from build123d import *

# Parameters (mm, degrees)
BOSS_EXTRUDE1_DEPTH                      = 3
MIRROR1_AT_THE_SECOND_PLANE_COPY_1_DEPTH = 3
SKETCH2_R                                = 8.5
SKETCH2_R_2                              = 4.75
CUT_EXTRUDE1_DEPTH                       = 108.522090753
SKETCH3_R                                = 1.6
CUT_EXTRUDE2_DEPTH                       = 108.522090753
CHAMFER1_SIZE                            = 1.5


with BuildPart() as part:
    # Sketch1 → Boss-Extrude1 (new body)
    with BuildSketch(Plane(origin=(0, 0, 0), x_dir=(1, 0, 0), z_dir=(0, 1, 0))):
        Polygon((-76, -73), (-59.111111111, -73), (-59.111111111, -76), (-42.222222222, -76), (-42.222222222, -73), (-25.333333333, -73), (-25.333333333, -76), (-8.444444444, -76), (-8.444444444, -73), (0, -73), (0, 0), (-76, 0), (-76, -8.444444444), (-73, -8.444444444), (-73, -25.333333333), (-76, -25.333333333), (-76, -42.222222222), (-73, -42.222222222), (-73, -59.111111111), (-76, -59.111111111), align=None)
    boss_extrude1 = extrude(amount=BOSS_EXTRUDE1_DEPTH)



with BuildPart() as mirror1_1:
    # Mirror1: Boss-Extrude1 across plane
    add(boss_extrude1.mirror(Plane(origin=(0, 0, 0), x_dir=(0, 0, 1), z_dir=(1, 0, 0))))


with BuildPart() as part_1:
    add(part.part)

    add(mirror1_1.part)  # Mirror1 at the second plane merges Mirror1_1
    # Mirror1 at the second plane: Boss-Extrude1 across plane
    add(boss_extrude1.mirror(Plane.XY))

    # Mirror1 at the second plane copy 1 sketc → Mirror1 at the second plane copy 1 (add)
    with BuildSketch(Plane(origin=(0, 0, 0), x_dir=(-1, 0, 0), z_dir=(0, 1, 0))):
        Polygon((-76, -73), (-59.111111111, -73), (-59.111111111, -76), (-42.222222222, -76), (-42.222222222, -73), (-25.333333333, -73), (-25.333333333, -76), (-8.444444444, -76), (-8.444444444, -73), (0, -73), (0, 0), (-76, 0), (-76, -8.444444444), (-73, -8.444444444), (-73, -25.333333333), (-76, -25.333333333), (-76, -42.222222222), (-73, -42.222222222), (-73, -59.111111111), (-76, -59.111111111), align=None)
    extrude(amount=MIRROR1_AT_THE_SECOND_PLANE_COPY_1_DEPTH)

    # Sketch2 → Cut-Extrude1 (cut, through all)
    with BuildSketch(Plane(origin=(0, 3, 0), x_dir=(1, 0, 0), z_dir=(0, 1, 0))):
        with Locations(Location((-13, -13.96, 0), (0, 0, 270))):
            Circle(SKETCH2_R)
        with Locations(Location((13, -13.96, 0), (0, 0, 270))):
            Circle(SKETCH2_R)
        with Locations(Location((0, -32.73, 0), (0, 0, 270))):
            Circle(SKETCH2_R_2)
    extrude(amount=-CUT_EXTRUDE1_DEPTH, mode=Mode.SUBTRACT)

    # Sketch3 → Cut-Extrude2 (cut, through all)
    with BuildSketch(Plane(origin=(0, 3, 0), x_dir=(1, 0, 0), z_dir=(0, 1, 0))):
        with Locations(Location((-18.3, -65.5, 0), (0, 0, 270))):
            Circle(SKETCH3_R)
        with Locations(Location((18.3, -65.5, 0), (0, 0, 270))):
            Circle(SKETCH3_R)
    extrude(amount=-CUT_EXTRUDE2_DEPTH, mode=Mode.SUBTRACT)

    # Chamfer1
    chamfer1_edges = [part_1.edges().sort_by_distance(p)[0] for p in [
        (-18.3, 3, 63.9),
        (18.3, 3, 63.9),
    ]]
    chamfer(chamfer1_edges, length=CHAMFER1_SIZE)


solid = part_1.part
The listing builds one solid part. Answer for the finished solid, in the listing's coordinates (mm). Give positions to 0.01 mm unless a question says otherwise; leave off trailing zeros. Write each loop counter-clockwise with the first axis right and the second up, starting at its lowest first coordinate (ties: lowest second). Pieces come first, ordered by that corner, then holes.
Item 1: Section A-A, the plane z = 13.96 is taken. Write down the section's boundary in (x, y).
Item 2: Determine the mould class of faces 1 (the flat face through (1, 0, 1)), 2 (the cylindrical face through (-10.45, 1.52, 22.07)) for opening direction X: released by +X, released by -X, zero draft, split by the parting line, or undercut.
Item 3: Section D-D, the plane x = -62.5 is taken. Write down the section's boundary in (y, z), plus the area to 3 significant figures.
Item 4: Section C-C, the plane y = 0.5 is taken. Count the separate pieces of the cut face and the enclosed holes in it, plus the area to 3 significant figures.
Item 5: Find the intervals of material crossed by line 1 along X through (y, z) = (1.25, 65.5); line 2 along X through (y, z) = (1.5, 13.96); line 3 along X through (y, z) = (1.6, 32.73), in increasing order.
Item 6: Flat-ended cylindrical pins translate along their axes: P1, Ø0.9, axis at y = 2, z = -49, coming from the +X side; P2, Ø1.5, axis at y = 1.5, z = 74, coming from the +X side; P3, Ø0.9, axis at x = 35, y = 2, coming from the +Z side. Find the tip coordinate at first contact, or state that the pin passes through.
Item 7: Section B-B, the plane x = 0 is taken. Write down the section's boundary in (y, z).
Completed:
1. outline: (-73, 0) - (-21.5, 0) - (-21.5, 3) - (-73, 3) - close; (-4.5, 0) - (4.5, 0) - (4.5, 3) - (-4.5, 3) - close; (21.5, 0) - (73, 0) - (73, 3) - (21.5, 3) - close
2. face 1: zero draft
2. face 2: undercut
3. outline: (0, -73) - (3, -73) - (3, 73) - (0, 73) - close
3. area: 438 mm2
4. separate pieces: 1
4. enclosed holes: 5
4. area: 21,700 mm2
5. line 1: x = -76 to -19.9, -16.7 to 16.7, 19.9 to 76
5. line 2: x = -73 to -21.5, -4.5 to 4.5, 21.5 to 73
5. line 3: x = -76 to -4.75, 4.75 to 76
6. P1: stops at x = 73
6. P2: stops at x = 59.11
6. P3: stops at z = 73
7. outline: (0, -73) - (3, -73) - (3, 27.98) - (0, 27.98) - close; (0, 37.48) - (3, 37.48) - (3, 73) - (0, 73) - close
